from build123d import *

# Parameters (mm, degrees)
SKETCH1_W               = 57.15
SKETCH1_H               = 25.4
BOSS_EXTRUDE1_DEPTH     = 12.7
BOSS_EXTRUDE3_DEPTH     = 12.7
CUT_EXTRUDE1_DEPTH      = 26.4
CUT_EXTRUDE2_DEPTH      = 26.4
FILLET1_R               = 6.35
SKETCH7_W               = 12.7
SKETCH7_H               = 2.286
BOSS_EXTRUDE4_DEPTH     = 25.4
SKETCH6_R               = 2.15
CUT_EXTRUDE3_DEPTH      = 14.413396589
CUT_EXTRUDE3_DEPTH_BACK = 12.4837718


with BuildPart() as part:
    # Sketch1 → Boss-Extrude1 (new body)
    with BuildSketch(Plane(origin=(0, 0, 0), x_dir=(1, 0, 0), z_dir=(0, 1, 0))):
        with Locations((14.605, 0)):
            Rectangle(SKETCH1_W, SKETCH1_H)
        with BuildLine():
            Line((-4.250232935, 8.382), (4.250232935, 8.382))
            ThreePointArc((4.250232935, 8.382), (9.398, 0), (4.250232935, -8.382))
            Line((4.250232935, -8.382), (-4.250232935, -8.382))
            ThreePointArc((-4.250232935, -8.382), (-9.398, 0), (-4.250232935, 8.382))
        make_face(mode=Mode.SUBTRACT)
        with BuildLine():
            Line((24.959767065, 8.382), (33.460232935, 8.382))
            ThreePointArc((33.460232935, 8.382), (38.608, 0), (33.460232935, -8.382))
            Line((33.460232935, -8.382), (24.959767065, -8.382))
            ThreePointArc((24.959767065, -8.382), (19.812, 0), (24.959767065, 8.382))
        make_face(mode=Mode.SUBTRACT)
    extrude(amount=BOSS_EXTRUDE1_DEPTH)

    # Sketch3 → Boss-Extrude3 (add)
    with BuildSketch(Plane.XZ):
        Polygon((-13.97, 12.7), (43.18, 12.7), (43.18, 5.6417718), (32.093467094, 5.6417718), (26.326532906, 5.6417718), (2.727750443, 5.6417718), (-2.727750443, 5.6417718), (-13.97, 5.6417718), align=None)
        with BuildLine():
            Line((43.18, -1.2162282), (43.18, -12.7))
            Line((43.18, -12.7), (-13.97, -12.7))
            Line((-13.97, -12.7), (-13.97, -1.2162282))
            Line((-13.97, -1.2162282), (-5.584085777, -1.2162282))
            ThreePointArc((-5.584085777, -1.2162282), (0, -5.715), (5.584085777, -1.2162282))
            Line((5.584085777, -1.2162282), (23.717811699, -1.2162282))
            ThreePointArc((23.717811699, -1.2162282), (29.21, -5.625241627), (34.702188301, -1.2162282))
            Line((34.702188301, -1.2162282), (43.18, -1.2162282))
        make_face()
    extrude(amount=BOSS_EXTRUDE3_DEPTH)

    # Sketch4 → Cut-Extrude1 (cut, through all)
    with BuildSketch(Plane.XZ.offset(12.7)):
        Polygon((-13.97, -6.9581141), (-13.97, -12.7), (0, -12.7), align=None)
        Polygon((29.21, -12.7), (43.18, -12.7), (43.18, -6.9581141), align=None)
        Polygon((43.18, 12.7), (43.18, 7.40632885), (29.21, 12.7), align=None)
        Polygon((0, 12.7), (-13.97, 6.751), (-13.97, 12.7), align=None)
    extrude(amount=-CUT_EXTRUDE1_DEPTH, mode=Mode.SUBTRACT)

    # Sketch5 → Cut-Extrude2 (cut, through all)
    with BuildSketch(Plane.XZ.offset(12.7)):
        Polygon((0, 12.7), (14.605, 6.35), (29.21, 12.7), align=None)
    extrude(amount=-CUT_EXTRUDE2_DEPTH, mode=Mode.SUBTRACT)

    # Fillet1
    fillet1_edges = [part.edges().sort_by_distance(p)[0] for p in [
        (0, 0, 12.7),
        (29.21, 0, 12.7),
        (29.21, 0, -12.7),
        (43.18, 0, -6.9581141),
        (-13.97, 0, -6.9581141),
        (0, 0, -12.7),
    ]]
    fillet(fillet1_edges, radius=FILLET1_R)

    # Sketch7 → Boss-Extrude4 (add)
    with BuildSketch(Plane.XZ.offset(12.7)):
        with Locations((14.605, 6.7847718)):
            Rectangle(SKETCH7_W, SKETCH7_H)
    extrude(amount=-BOSS_EXTRUDE4_DEPTH)

    # Sketch6 → Cut-Extrude3 (cut, two sides)
    with BuildSketch(Plane.XY.offset(-1.2162282)) as cut_extrude3_sk:
        with Locations((14.650948738, -6.35)):
            Circle(SKETCH6_R)
    extrude(amount=CUT_EXTRUDE3_DEPTH, mode=Mode.SUBTRACT)
    extrude(cut_extrude3_sk.sketch, amount=-CUT_EXTRUDE3_DEPTH_BACK, mode=Mode.SUBTRACT)


solid = part.part
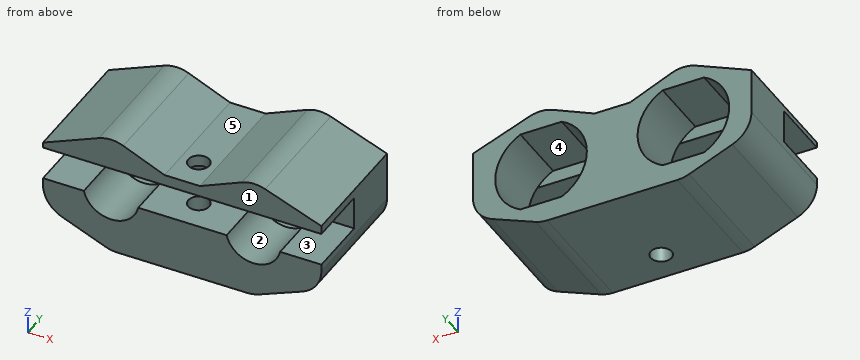
Here's how the part is built. I have some questions about the finished solid (model axes, mm). Face numbers are marked on the shaded views. A direction names the side the tool comes from. Coordinates: 2 decimals unless noted, no trailing zeros. Order: outer loops, then holes, each group sorted by start corner. A loop starts at its lowest first (then second) coordinate and runs counter-clockwise, first axis right, second up. Notation, with made-up numbers: (31, 16.25) - (57, 16.25) arc R22 cw to (57, 35.25) - close; hole circle Ø5 at (-6, 77). An arc over 180 degrees is marked (long way). Use CSV: the item, a comma, the result in double quotes. Start each with the question number.
1. Suppose I cut it at B-B on x = 20.5. List the corners of the cut face in (y, z) for me.
2. Suppose I cut it at C-C on y = -6.35. Give the number of separate pieces and of enclosed holes in the cut face, then the cut area to 3 significant figures.
3. Suppose I cut it at A-A on y = 8. List the corners of the cut face in (x, z) for me, then the cut area to 3 significant figures.
4. For the marked faces 1, 2, 3, 4 and 5, which set-ups out of +Z, -Z, +X, -X, +Y, -Y let a thin tool reach every point of the face, with its end or its side?
5. Suppose I cut it at D-D on z = 1.25. List the corners of the cut face in (x, y) for me.
6. Please list where these lines run through material, in increasing order: line 1 (X direction, y = 9.5, z = -4.75); line 2 (X direction, y = -4, z = -4.5); line 3 (Y direction, x = -4.5, z = -3.75). Write a range as from..to.
7. I'm going to push flat-ended pins straight in: pin 1 (1.4 mm diameter, centred on x = 32.5, z = 7, fed in from +Y); pin 2 (3.5 mm diameter, centred on x = 14, y = 1.5, fed in from +Z); pin 3 (2.5 mm diameter, centred on x = 14.65, y = -6.35, fed in from +Z); pin 4 (1.9 mm diameter, centred on x = 41.5, z = 3, fed in from -Y). Where does each tip first touch, or does it pass through?
Output:
1,outline,"(-12.7, -12.7) - (12.7, -12.7) - (12.7, -3.53) - (0, -3.53) - (0, -1.22) - (-12.7, -1.22) - close; (-12.7, 5.64) - (0, 5.64) - (0, 3.53) - (12.7, 3.53) - (12.7, 8.91) - (-12.7, 8.91) - close"
2,separate pieces,"4"
2,enclosed holes,"0"
2,area,"673 mm2"
3,outline,"(-13.97, -2.7) arc R6.35 ccw to (-10.03, -8.58) - (-1.16, -12.22) arc R6.35 ccw to (1.25, -12.7) - (27.96, -12.7) arc R6.35 ccw to (30.37, -12.22) - (39.24, -8.58) arc R6.35 ccw to (43.18, -2.7) - (43.18, 7.41) - (31.62, 11.79) arc R6.35 ccw to (26.84, 11.67) - (18.23, 7.93) - (10.98, 7.93) - (2.51, 11.61) arc R6.35 ccw to (-2.51, 11.63) - (-13.97, 6.75) - close; hole (-4.25, -8.38) - (4.25, -8.38) arc R9.4 ccw to (4.25, 8.38) - (-4.25, 8.38) arc R9.4 ccw to start; hole (24.96, -8.38) - (33.46, -8.38) arc R9.4 ccw to (33.46, 8.38) - (24.96, 8.38) arc R9.4 ccw to start"
3,area,"666 mm2"
4,face 1,"+Z, -Z, +X, -X, -Y"
4,face 2,"+Y, -Y"
4,face 3,"+X, -X, -Y"
4,face 4,"+Y"
4,face 5,"+Z, +Y, -Y"
5,outline,"(-13.97, 0) - (-9.31, 0) - (-9.31, 12.7) - (-13.97, 12.7) - close; (9.31, 0) - (19.9, 0) - (19.9, 12.7) - (9.31, 12.7) - close; (38.52, 0) - (43.18, 0) - (43.18, 12.7) - (38.52, 12.7) - close"
6,line 1,"x = -13.63..-8.11, 8.11..21.1, 37.32..42.84"
6,line 2,"x = -13.71..-3.52, 3.52..25.83, 32.59..42.92"
6,line 3,"y = -12.7..0"
7,pin 1,"stops at y = 0"
7,pin 2,"stops at z = 7.93"
7,pin 3,"passes through"
7,pin 4,"stops at y = 0"
